Verification items for the finished model (mm, model axes). Give positions to 0.01 mm unless a question says otherwise; leave off trailing zeros. Write each loop counter-clockwise with the first axis right and the second up, starting at its lowest first coordinate (ties: lowest second). Pieces come first, ordered by that corner, then holes. Notation, with made-up numbers: (35.25, 73.5) -> (46.25, 73.5) arc R27 ccw to (46.25, 91.5) -> close; hole circle Ø10 at (-1.5, 47.25). An arc over 180 degrees is marked (long way). Answer as CSV lines item,"result". Start each with the question number.
1) Gauge pin test, flat end, axial feed: pin 1 Ø1.8 at (x, z) = (10, 46.5) entering from +Y. Record the tip position at first contact, or that the pin passes through.
2) Material ranges on L1, parallel to Z at x = 10, y = -4; L2, parallel to X at y = -19, z = 114; L3, parallel to Y at x = 1.75, z = 172, recorded low to high.
3) Sectioned sample at B-B on z = 129. Record the cut outline in (x, y).
4) Sectioned sample at A-A on x = 10. Record the cut outline in (y, z).
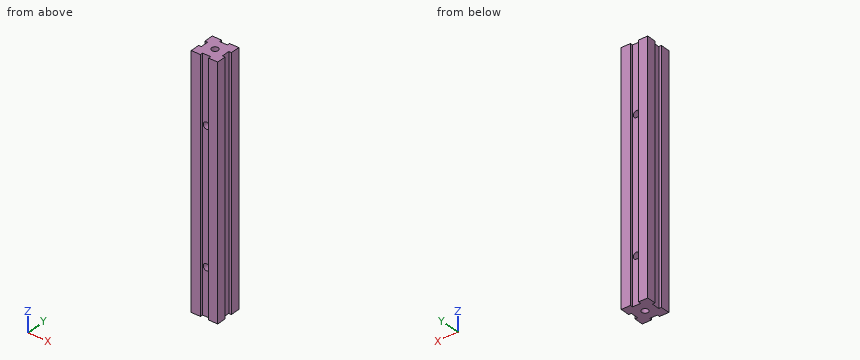
```python
from build123d import *

# Parameters (mm, degrees)
SKETCH_1_R          = 2.5
EXTRUDE_1_DEPTH     = 185
SKETCH_2_R          = 2.5
CUT_EXTRUDE_1_DEPTH = 188.149672722


with BuildPart() as part:
    # 草图1 → 凸台-拉伸1 (new body)
    with BuildSketch(Plane.XY):
        Polygon((0, -13), (0, -20), (7, -20), (7, -18), (13, -18), (13, -20), (20, -20), (20, -13), (18, -13), (18, -7), (20, -7), (20, 0), (13, 0), (13, -2), (7, -2), (7, 0), (0, 0), (0, -7), (2, -7), (2, -13), align=None)
        with Locations((10, -10)):
            Circle(SKETCH_1_R, mode=Mode.SUBTRACT)
    extrude(amount=EXTRUDE_1_DEPTH)

    # 草图2 → 切除-拉伸1 (cut, through all)
    with BuildSketch(Plane(origin=(0, 0, 0), x_dir=(1, 0, 0), z_dir=(0, 1, 0))):
        with Locations(Location((10, -35, 0), (0, 0, 270))):
            Circle(SKETCH_2_R)
        with Locations(Location((10, -135, 0), (0, 0, 270))):
            Circle(SKETCH_2_R)
    extrude(amount=-CUT_EXTRUDE_1_DEPTH, mode=Mode.SUBTRACT)


solid = part.part
```
Ans:
1,pin 1,"stops at y = -2"
2,L1,"z = 0 to 32.5, 37.5 to 132.5, 137.5 to 185"
2,L2,"x = 0 to 7, 13 to 20"
2,L3,"y = -20 to -13, -7 to 0"
3,outline,"(0, -20) -> (7, -20) -> (7, -18) -> (13, -18) -> (13, -20) -> (20, -20) -> (20, -13) -> (18, -13) -> (18, -7) -> (20, -7) -> (20, 0) -> (13, 0) -> (13, -2) -> (7, -2) -> (7, 0) -> (0, 0) -> (0, -7) -> (2, -7) -> (2, -13) -> (0, -13) -> close; hole circle Ø5 at (10, -10)"
4,outline,"(-18, 0) -> (-12.5, 0) -> (-12.5, 32.5) -> (-18, 32.5) -> close; (-18, 37.5) -> (-12.5, 37.5) -> (-12.5, 132.5) -> (-18, 132.5) -> close; (-18, 137.5) -> (-12.5, 137.5) -> (-12.5, 185) -> (-18, 185) -> close; (-7.5, 0) -> (-2, 0) -> (-2, 32.5) -> (-7.5, 32.5) -> close; (-7.5, 37.5) -> (-2, 37.5) -> (-2, 132.5) -> (-7.5, 132.5) -> close; (-7.5, 137.5) -> (-2, 137.5) -> (-2, 185) -> (-7.5, 185) -> close"
